Read the model definition and answer for the solid it produces. Units are mm, in the model's axes. Face numbers are marked on the shaded views. A direction names the side the tool comes from. Give positions to 0.01 mm unless a question says otherwise; leave off trailing zeros. Order: outer loops, then holes, each group sorted by start corner. A loop starts at its lowest first (then second) coordinate and runs counter-clockwise, first axis right, second up. Notation, with made-up numbers: (42, 21.25) - (69, 21.25) arc R23 ccw to (69, 54.25) - close; hole circle Ø6 at (34.25, -9.5). An arc over 180 degrees is marked (long way). Write each question's results on one line, items separated by ' | '. Start each with the question number.
Q1. For a pull along Y with two mould halves and no side action, classify the marked faces 6, 7 and 8 as +Y half, -Y half, draft (parallel to the pull), parting line (faces both ways), or undercut.
Q2. Find section B-B on y = 7. Give the vertices of the cut face in (x, z), and give its area (3 significant figures).
Q3. Find section D-D on z = 5. Give the vertices of the cut face in (x, y).
Q4. Find section A-A on z = 0. Give the vertices of the cut face in (x, y), and give its area (3 significant figures).
Q5. Flat-ended cylindrical pins translate along their axes: P1, Ø2.5, axis at y = 0, z = -7, coming from the +X side; P2, Ø5, axis at x = 2, z = 13, coming from the +Y side; P3, Ø1.6, axis at y = 7, z = 0, coming from the +X side; P4, Ø6, axis at x = 7, y = -8.5, coming from the -Z side. Find the tip coordinate at first contact, or state that the pin passes through.
Q6. Find the intervals of material crossed by line 1 along Y through (x, z) = (7.85, 0); line 2 along Y through (x, z) = (3.05, 7); line 3 along Y through (x, z) = (8.5, -3), in increasing order. Write a range as from..to.
Q7. Find section C-C on x = 1. Count the separate pieces of the cut face and the enclosed holes in it, and give its area (3 significant figures).
Q8. A tool of negligible diameter and unlimited length cuts with its end or side. For the marked faces 1, 2, 3, 4 and 5, from which of +Z, -Z, +X, -X, +Y, -Y can it reach the whole face along a straight path? Write none if from no direction.
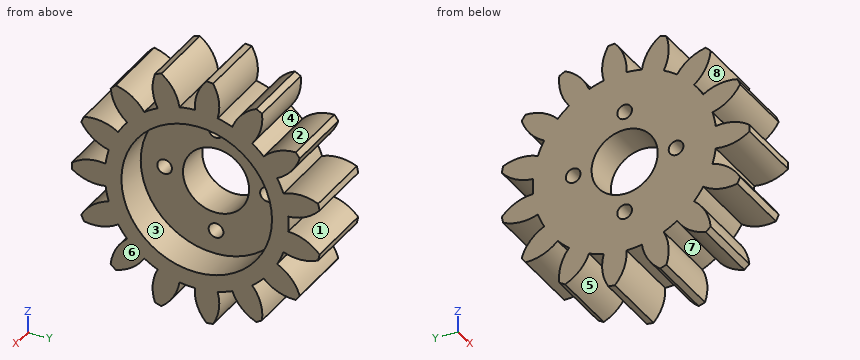
from build123d import *

# Parameters (mm, degrees)
BASPROSKE_W         = 10
BASPROSKE_H         = 17
TOOTHCUT_DEPTH      = 27.038433133
TEETHCUTS_COUNT     = 15
BORSKE_R            = 10.25
BORE_DEPTH          = 10
SKETCH1_R           = 10.25
SKETCH1_R_2         = 1
SKETCH1_R_3         = 4.5
BOSS_EXTRUDE1_DEPTH = 5


with BuildPart() as part:
    # BasProSke → Base-Revolve (revolve)
    with BuildSketch(Plane(origin=(0, 0, 0), x_dir=(1, 0, 0), z_dir=(0, 1, 0)), mode=Mode.PRIVATE) as base_revolve_sk:
        with Locations((5, 8.5)):
            Rectangle(BASPROSKE_W, BASPROSKE_H)
    revolve(base_revolve_sk.sketch.rotate(Axis((-10, 0, 0), (1, 0, 0)), 180), axis=Axis((-10, 0, 0), (1, 0, 0)))

    # TooCutSke → ToothCut (cut, through all)
    with BuildSketch(Plane(origin=(0, 0, 0), x_dir=(0, 0, -1), z_dir=(1, 0, 0))):
        with BuildLine():
            ThreePointArc((1.050056448, 12.454813626), (0, 12.499), (-1.050056448, 12.454813626))
            ThreePointArc((-1.050056448, 12.454813626), (-1.638118106, 14.809604533), (-3.110934279, 16.73876737))
            ThreePointArc((-3.110934279, 16.73876737), (0, 17.0254), (3.110934279, 16.73876737))
            ThreePointArc((3.110934279, 16.73876737), (1.638118106, 14.809604533), (1.050056448, 12.454813626))
        make_face()
    toothcut = extrude(amount=TOOTHCUT_DEPTH, mode=Mode.SUBTRACT)

    # TeethCuts: ToothCut ×15 about axis
    teethcuts_axis = Axis((0, 0, 0), (1, 0, 0))
    for i in range(1, TEETHCUTS_COUNT):
        add(toothcut.rotate(teethcuts_axis, i * 360 / TEETHCUTS_COUNT), mode=Mode.SUBTRACT)

    # BorSke → Bore (cut, symmetric)
    with BuildSketch(Plane(origin=(0, 0, 0), x_dir=(0, 0, -1), z_dir=(1, 0, 0))):
        with Locations(Location((0, 0, 0), (0, 0, 180))):
            Circle(BORSKE_R)
    extrude(amount=BORE_DEPTH, both=True, mode=Mode.SUBTRACT)

    # Sketch1 → Boss-Extrude1 (add)
    with BuildSketch(Plane(origin=(0, 0, 0), x_dir=(0, 0, -1), z_dir=(1, 0, 0))):
        with Locations(Location((0, 0, 0), (0, 0, 180))):
            Circle(SKETCH1_R)
        with Locations((7, 0)):
            Circle(SKETCH1_R_2, mode=Mode.SUBTRACT)
        with Locations((-7, 0)):
            Circle(SKETCH1_R_2, mode=Mode.SUBTRACT)
        with Locations((0, 7)):
            Circle(SKETCH1_R_2, mode=Mode.SUBTRACT)
        with Locations((0, -7)):
            Circle(SKETCH1_R_2, mode=Mode.SUBTRACT)
        Circle(SKETCH1_R_3, mode=Mode.SUBTRACT)
    extrude(amount=BOSS_EXTRUDE1_DEPTH)


solid = part.part
Working result:
1) face 6: draft | face 7: undercut | face 8: -Y half
2) outline: (0, -14.33) - (10, -14.33) - (10, -7.49) - (5, -7.49) - (5, -1) - (0, -1) - close; (0, 1) - (5, 1) - (5, 7.49) - (10, 7.49) - (10, 14.33) - (0, 14.33) - close | area: 202 mm²
3) outline: (0, -14.52) - (10, -14.52) - (10, -8.95) - (5, -8.95) - (5, 8.95) - (10, 8.95) - (10, 11.46) - (0, 11.46) - close
4) outline: (0, -17) - (10, -17) - (10, -10.25) - (5, -10.25) - (5, -8) - (0, -8) - close; (0, -6) - (5, -6) - (5, -4.5) - (0, -4.5) - close; (0, 4.5) - (5, 4.5) - (5, 6) - (0, 6) - close; (0, 8) - (5, 8) - (5, 10.25) - (10, 10.25) - (10, 12.5) - (0, 12.5) - close | area: 127 mm²
5) P1: x = 5 | P2: y = 8.93 | P3: through | P4: z = -16.09
6) line 1: -17..-10.25, 10.25..12.5 | line 2: -15.49..-11.67, -10.35..-1, 1..12.37 | line 3: -12.13..-9.8, 9.8..16.64
7) separate pieces: 1 | enclosed holes: 5 | area: 597 mm²
8) face 1: +X, -X, +Y | face 2: +Z, +X, -X | face 3: +X | face 4: +X, -X | face 5: -Z, +X, -X
